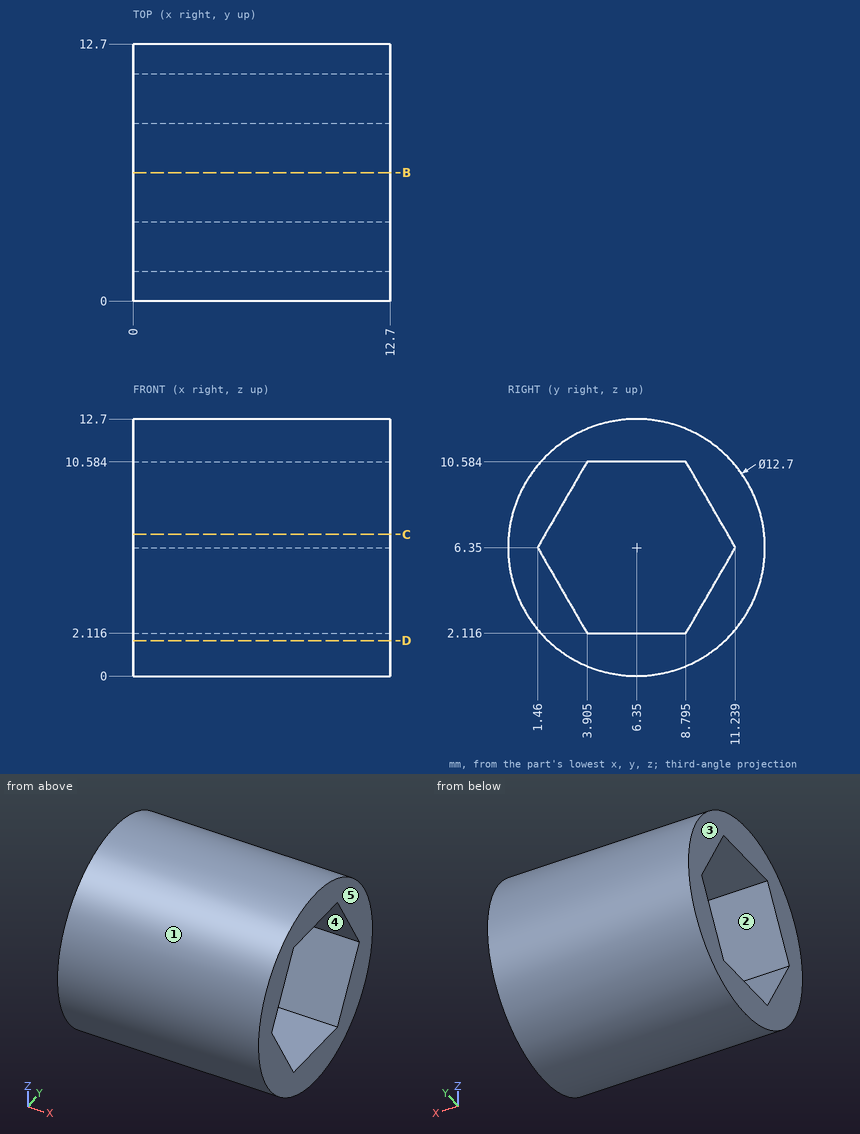
Design review of the part shown in the three views and the two pictorial views. Dimensions are in mm from the part's minimum x, y and z. A direction names the side the tool comes from. Give positions to 0.01 mm unless a question says otherwise; leave off trailing zeros. Loops run counter-clockwise (first coordinate to the right, second up) from the corner with the lowest first, then second, coordinate; pieces in that order, holes last. Notation, with made-up numbers: (-9.5, 63.25) -> (48.5, 63.25) arc R31 ccw to (48.5, 101.25) -> close; hole circle Ø11 at (-22.5, -15). An arc over 180 degrees is marked (long way). One line per question, with ' | ' between items.
1) To check wall thickness, follow probe 1 along Y at (x, z) = (7, 8.75) (1 decimal); probe 2 along Z at (x, y) = (1.75, 3.5) (1 decimal); probe 3 along Y at (x, z) = (7.25, 7.75) (1 decimal). State the ranges of each line that lie inside material, in increasing order.
Resolved:
probe 1: y = 0.5 to 2.8, 9.9 to 12.2 | probe 2: z = 0.7 to 2.8, 9.9 to 12 | probe 3: y = 0.2 to 2.3, 10.4 to 12.5
2) For the marked faces 4 and 5, list the 3-axis set-ups (+Z, -Z, +X, -X, +Y, -Y) from which the entire face can be reached by the end or side of a thin tool; tool diameter is ignored.
Resolved:
face 4: +X, -X | face 5: +Z, -Z, +X, +Y, -Y
3) Insertion check: pin 1 Ø5 at (x, y) = (3.5, 10.5) entering from +Z; pin 2 Ø4 at (x, z) = (3.5, 4) entering from -Y; pin 3 Ø2 at (x, y) = (1.5, 3) entering from +Z. Each pin has a flat end and moves straight along its axis. Give the tip position at first contact, or say it passes through.
Resolved:
pin 1: stops at z = 12.48 | pin 2: stops at y = 0.01 | pin 3: stops at z = 12.25
4) The part is to be moulded in two halves that separate along Z. For the marked faces 1, 2 and 3, say which applies: +Z half, -Z half, draft (parallel to the pull), parting line (faces both ways), or undercut.
Resolved:
face 1: parting line | face 2: undercut | face 3: draft
5) We need section D-D (z = 1.75). Write out the cut boundary in (x, y).
Resolved:
outline: (0, 1.97) -> (12.7, 1.97) -> (12.7, 10.73) -> (0, 10.73) -> close
6) We need section C-C (z = 7). Write out the cut boundary in (x, y) (1 decimal).
Resolved:
outline: (0, 0) -> (12.7, 0) -> (12.7, 1.8) -> (0, 1.8) -> close; (0, 10.9) -> (12.7, 10.9) -> (12.7, 12.7) -> (0, 12.7) -> close
7) We need section B-B (y = 6.35). Write out the cut boundary in (x, z) (1 decimal).
Resolved:
outline: (0, 0) -> (12.7, 0) -> (12.7, 2.1) -> (0, 2.1) -> close; (0, 10.6) -> (12.7, 10.6) -> (12.7, 12.7) -> (0, 12.7) -> close
